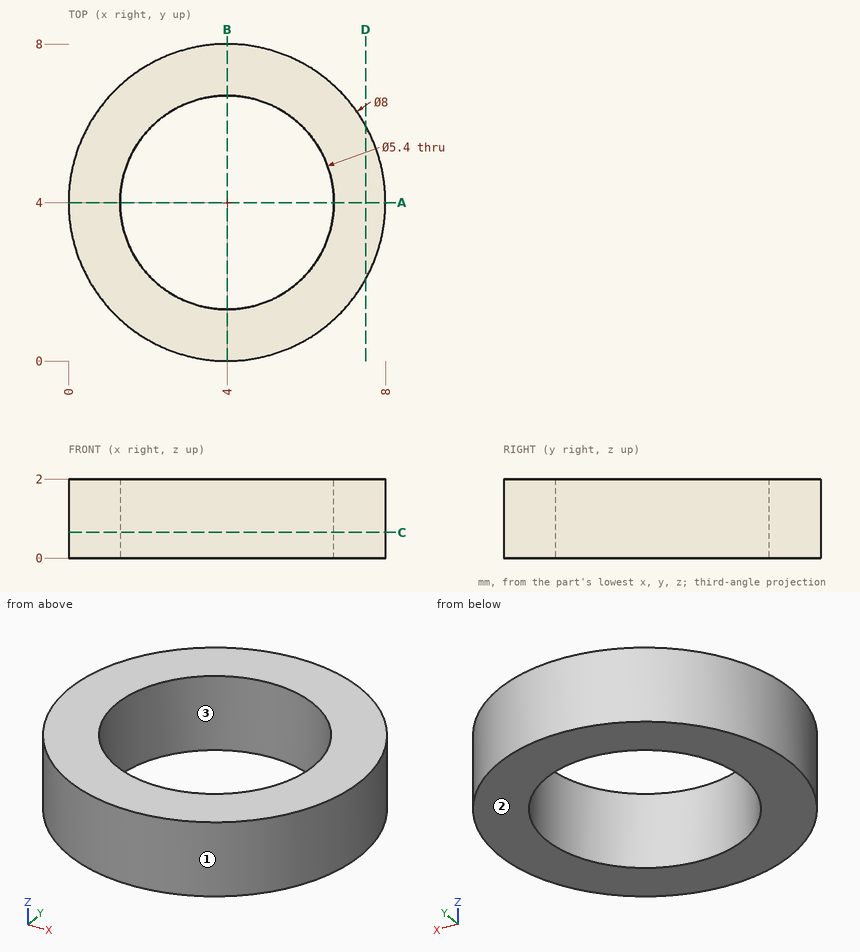
Answer from the drawing. Dimensions are ordinates in mm from the lowest x, y and z of the part. Round coordinates to 2 decimals unless told otherwise and drop trailing zeros. Write each loop counter-clockwise with the first axis right and the second up, starting at its lowest first coordinate (ties: lowest second). Pieces come first, ordered by that corner, then holes. Notation, with made-up numbers: M -35.75,25.5 L 12.25,25.5 A6 cw 12.25,31.5 Z; hole C 56.25,41 d1. An arc over 180 degrees is marked long. Write each question's results on one line, items separated by ' | '. Start each with the question number.
Item 1: A cutting plane is placed at A-A on y = 4. Write down the section's boundary in (x, z), and give its area (3 significant figures).
Item 2: A cutting plane is placed at C-C on z = 0.65. Write down the section's boundary in (x, y).
Item 3: For a pull along Y with two mould halves and no side action, classify the marked faces 1, 2 and 3 as pulls with the +Y half, pulls with the -Y half, needs draft (parallel to the pull), parting line crosses it, or undercut.
Item 4: A cutting plane is placed at D-D on x = 7.5. Write down the section's boundary in (y, z).
Item 5: Straight lines are drawn through the part: L1, parallel to Y at x = 4, z = 1.85; L2, parallel to X at y = 2.75, z = 0.5; L3, parallel to Y at x = 2.5, z = 0.35 (3 decimals). For each, find the intervals that lie inside material, in ascending order. Write a range as [from, to].
Check sheet entries:
1) outline: M 0,0 L 1.3,0 L 1.3,2 L 0,2 Z; M 6.7,0 L 8,0 L 8,2 L 6.7,2 Z | area: 5.20 mm²
2) outline: C 4,4 d8; hole C 4,4 d5.4
3) face 1: parting line crosses it | face 2: needs draft | face 3: undercut
4) outline: M 2.06,0 L 5.94,0 L 5.94,2 L 2.06,2 Z
5) L1: [0, 1.3], [6.7, 8] | L2: [0.2, 1.61], [6.39, 7.8] | L3: [0.292, 1.755], [6.245, 7.708]
